Autodesk Inventor part; units mm, degrees
sketch "Sketch1" plane through (0, 0, 0) normal (0, 0, 1) x (1, 0, 0)
  line L0 (0, 2.8582) -> (0, -2.8582) construction
  line L1 (-5.7775, 0) -> (5.7775, 0) construction
  circle A0 centre (0, 0) radius 35.629
  circle A1 centre (0, 0) radius 4
  line L2 (0, 4) -> (0, 7)
  line L3 (0, 7) -> (0, 21)
  line L4 (0, 21) -> (5, 21)
  line L5 (5, 21) -> (8, 21)
  line L6 (8, 21) -> (0, 7)
  line L7 (0, 21) -> (-8, 21)
  line L8 (-8, 21) -> (0, 7)
  line L9 (0, -4) -> (0, -7)
  line L10 (0, -7) -> (0, -21)
  line L11 (0, -21) -> (8, -21)
  line L12 (8, -21) -> (0, -7)
  line L13 (0, -21) -> (-8, -21)
  line L14 (-8, -21) -> (0, -7)
  line L15 (0, 0) -> (2.5981, 1.5)
  line L16 (0, 0) -> (3, 0) construction
  line L17 (2.5981, 1.5) -> (3.4641, 2)
  line L18 (3.4641, 2) -> (6.0622, 3.5)
  line L19 (6.0622, 3.5) -> (18.1865, 10.5)
  line L20 (18.1865, 10.5) -> (14.1865, 17.4282)
  line L21 (14.1865, 17.4282) -> (6.0622, 3.5)
  line L22 (18.1865, 10.5) -> (22.1865, 3.5718)
  line L23 (22.1865, 3.5718) -> (6.0622, 3.5)
  line L24 (0, 0) -> (8, 0) construction
  line L25 (0, 0) -> (3.4641, -2)
  line L26 (0, 0) -> (4, 0) construction
  line L27 (3.4641, -2) -> (6.0622, -3.5)
  line L28 (6.0622, -3.5) -> (18.1865, -10.5)
  line L29 (18.1865, -10.5) -> (14.1865, -17.4282)
  line L30 (14.1865, -17.4282) -> (6.0934, -3.518)
  line L31 (18.1865, -10.5) -> (22.0919, -3.518)
  line L32 (22.0919, -3.518) -> (6.0934, -3.518)
  line L33 (0, 0) -> (-2.5981, 1.5)
  line L34 (0, 0) -> (3, 0) construction
  line L35 (-2.5981, 1.5) -> (-3.4641, 2)
  line L36 (-3.4641, 2) -> (-6.0622, 3.5)
  line L37 (-6.0622, 3.5) -> (-18.1865, 10.5)
  line L38 (-18.1865, 10.5) -> (-14.1865, 17.4282)
  line L39 (-14.1865, 17.4282) -> (-6.0622, 3.5)
  line L40 (-18.1865, 10.5) -> (-22.1865, 3.5718)
  line L41 (-22.1865, 3.5718) -> (-6.0622, 3.5)
  line L42 (0, 0) -> (-6.0622, -3.5)
  line L43 (0, 0) -> (7, 0) construction
  line L44 (-6.0622, -3.5) -> (-18.1865, -10.5)
  line L45 (-18.1865, -10.5) -> (-14.1865, -17.4282)
  line L46 (-14.1865, -17.4282) -> (-6.0622, -3.5)
  line L47 (-18.1865, -10.5) -> (-22.1865, -3.5718)
  line L48 (-22.1865, -3.5718) -> (-6.0622, -3.5)
  dimension "d0" = 71.258
  dimension "d1" = 8
  dimension "d2" = 3
  dimension "d3" = 14
  dimension "d4" = 5
  dimension "d5" = 3
  dimension "d6" = 8
  dimension "d7" = 3
  dimension "d8" = 14
  dimension "d9" = 8
  dimension "d10" = 8
  dimension "d11" = 3
  dimension "d12" = 30
  dimension "d13" = 3
  dimension "d14" = 14
  dimension "d15" = 8
  dimension "d16" = 8
  dimension "d19" = 4
  dimension "d20" = 30
  dimension "d21" = 3
  dimension "d22" = 14
  dimension "d23" = 8
  dimension "d24" = 8
  dimension "d25" = 3
  dimension "d26" = 150
  dimension "d27" = 1
  dimension "d28" = 180
  dimension "d29" = 3
  dimension "d30" = 180
  dimension "d31" = 180
  dimension "d32" = 8
  dimension "d33" = 8
  dimension "d34" = 7
  dimension "d35" = 150
  dimension "d36" = 14
  dimension "d37" = 180
  dimension "d38" = 8
  dimension "d39" = 8
extrude "Extrusion1" add sketch "Sketch1" along normal blind 2
fillet "Fillet1" radius 2 18 edges at (14.1865, 17.4282, 1) (22.1865, 3.5718, 1) (6.0622, 3.5, 1) (22.0919, -3.518, 1) (14.1865, -17.4282, 1) (6.0934, -3.518, 1) (0, 7, 1) (-8, 21, 1) (8, 21, 1) (-6.0622, 3.5, 1) (-22.1865, 3.5718, 1) (-14.1865, 17.4282, 1) (-6.0622, -3.5, 1) (-14.1865, -17.4282, 1) (-22.1865, -3.5718, 1) (-8, -21, 1) (0, -7, 1) (8, -21, 1)
sketch "Sketch2" plane through (0, 0, 2) normal (0, 0, 1) x (1, 0, 0)
  circle A0 centre (0, 0) radius 3.05
  circle A1 centre (0, 0) radius 5
  dimension "d43" = 6.1
  dimension "d49" = 10
extrude "Extrusion2" add sketch "Sketch2" against normal blind 2
chamfer "Chamfer1" distance 1 angle 45 1 edges at (-35.629, 0, 2)
sketch "Sketch4" plane through (0, 0, 2) normal (0, 0, 1) x (1, 0, 0)
  circle A0 centre (0, 0) radius 3.05
  circle A1 centre (0, 0) radius 6
  dimension "d54" = 6.1
  dimension "d55" = 12
extrude "Extrusion4" add sketch "Sketch4" along normal blind 20
fillet "Fillet2" radius 2 1 edges at (-6, 0, 2)
properties part number "Wiel hout+spacer x 20mm" material "S235"
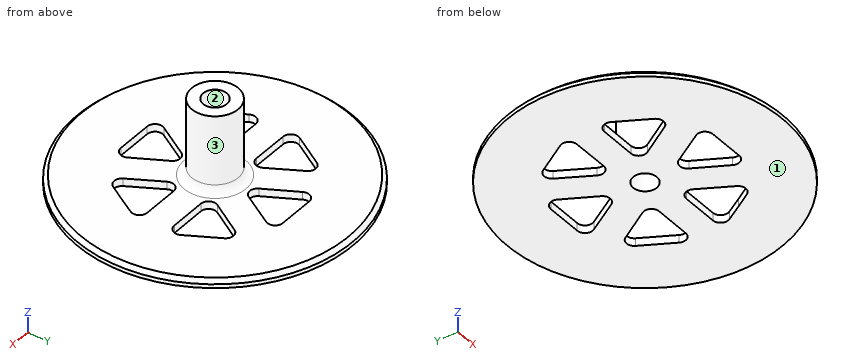
Geometry: final body of the model. Coordinates: model frame, mm. Face numbers are marked on the shaded views. Round coordinates to 2 decimals unless told otherwise and drop trailing zeros. Order: outer loops, then holes, each group sorted by start corner. A loop starts at its lowest first (then second) coordinate and runs counter-clockwise, first axis right, second up. Notation, with made-up numbers: (-24.75, 32.5) -> (-6.75, 32.5) arc R25 ccw to (-6.75, 57.5) -> close; hole circle Ø9 at (-7.75, 70). An arc over 180 degrees is marked (long way). Put each result on its own line as item: value. Start each with the question number.
Q1. Section A-A on x = 0. Return the cut outline in (y, z).
Q2. First-contact query: pin 1 (2 mm diameter, centred on x = -25.5, y = 11.5, fed in from -Z); pin 2 (12 mm diameter, centred on y = 9.5, z = 9.5, fed in from -X); pin 3 (2 mm diameter, centred on x = 14.5, z = 1, fed in from -Y); pin 4 (4 mm diameter, centred on x = 13.5, y = -19, fed in from +Z). Flat tips, straight axial feed; report the tip coordinate or a pass-through.
Q3. Pull-direction query (Y, two-part tool) for the marked faces 1, 2 and 3; classes: +Y half, -Y half, draft (parallel to the pull), parting line (faces both ways), or undercut.
Q4. Section B-B on y = 0. Return the cut outline in (x, z), and give its area (3 significant figures).
Q5. Line query: probe 1 along Y at (x, z) = (0, 10.25); probe 2 along Z at (x, y) = (17, 22.5). Output: solid intervals per line, ascending.
Q6. Section C-C on z = 8.5. Return the cut outline in (x, y).
Ans:
1. outline: (-35.63, 0) -> (-21, 0) -> (-21, 2) -> (-34.63, 2) -> (-35.63, 1) -> close; (-9.03, 0) -> (-3.05, 0) -> (-3.05, 22) -> (-6, 22) -> (-6, 4) arc R2 cw to (-8, 2) -> (-9.03, 2) -> close; (3.05, 0) -> (9.03, 0) -> (9.03, 2) -> (8, 2) arc R2 cw to (6, 4) -> (6, 22) -> (3.05, 22) -> close; (21, 0) -> (35.63, 0) -> (35.63, 1) -> (34.63, 2) -> (21, 2) -> close
2. pin 1: stops at z = 0
2. pin 2: stops at x = -4.87
2. pin 3: stops at y = -32.97
2. pin 4: stops at z = 2
3. face 1: draft
3. face 2: undercut
3. face 3: parting line
4. outline: (-35.63, 0) -> (-3.05, 0) -> (-3.05, 22) -> (-6, 22) -> (-6, 4) arc R2 cw to (-8, 2) -> (-34.63, 2) -> (-35.63, 1) -> close; (3.05, 0) -> (35.63, 0) -> (35.63, 1) -> (34.63, 2) -> (8, 2) arc R2 cw to (6, 4) -> (6, 22) -> (3.05, 22) -> close
4. area: 249 mm2
5. probe 1: y = -6 to -3.05, 3.05 to 6
5. probe 2: z = 0 to 2
6. outline: circle Ø12 at (0, 0); hole circle Ø6.1 at (0, 0)
